from build123d import *

# Parameters (mm, degrees)
BOSS_EXTRUDE1_DEPTH = 19.05
SKETCH3_W           = 5
SKETCH3_H           = 26.05
CUT_EXTRUDE2_DEPTH  = 3
BOSS_EXTRUDE2_DEPTH = 38.1
SKETCH5_R           = 1.5
CUT_EXTRUDE3_DEPTH  = 8.35
FILLET1_R           = 1


with BuildPart() as part:
    # Sketch1 → Boss-Extrude1 (new body, symmetric)
    with BuildSketch(Plane(origin=(0, 0, 0), x_dir=(0, 0, -1), z_dir=(1, 0, 0))):
        Polygon((0, 0), (-2, 0), (-2, 38), (-40, 38), (-40, 40), (0, 40), align=None)
    extrude(amount=BOSS_EXTRUDE1_DEPTH, both=True)

    # Sketch3 → Cut-Extrude2 (cut, through all)
    with BuildSketch(Plane.XY.offset(2)):
        with Locations((2.5, 17.394531681)):
            Rectangle(SKETCH3_W, SKETCH3_H)
        with Locations((-2.5, 17.394531681)):
            Rectangle(SKETCH3_W, SKETCH3_H)
        with BuildLine():
            Line((-9.525, 30.419531681), (-9.525, 20.419531681))
            ThreePointArc((-9.525, 20.419531681), (-8.025, 18.919531681), (-6.525, 20.419531681))
            Line((-6.525, 20.419531681), (-6.525, 30.419531681))
            ThreePointArc((-6.525, 30.419531681), (-8.025, 31.919531681), (-9.525, 30.419531681))
        make_face()
        with BuildLine():
            Line((-9.525, 14.369531681), (-9.525, 4.369531681))
            ThreePointArc((-9.525, 4.369531681), (-8.025, 2.869531681), (-6.525, 4.369531681))
            Line((-6.525, 4.369531681), (-6.525, 14.369531681))
            ThreePointArc((-6.525, 14.369531681), (-8.025, 15.869531681), (-9.525, 14.369531681))
        make_face()
        with BuildLine():
            ThreePointArc((9.525, 20.419531681), (8.025, 18.919531681), (6.525, 20.419531681))
            Line((6.525, 20.419531681), (6.525, 30.419531681))
            ThreePointArc((6.525, 30.419531681), (8.025, 31.919531681), (9.525, 30.419531681))
            Line((9.525, 30.419531681), (9.525, 20.419531681))
        make_face()
        with BuildLine():
            ThreePointArc((9.525, 4.369531681), (8.025, 2.869531681), (6.525, 4.369531681))
            Line((6.525, 4.369531681), (6.525, 14.369531681))
            ThreePointArc((6.525, 14.369531681), (8.025, 15.869531681), (9.525, 14.369531681))
            Line((9.525, 14.369531681), (9.525, 4.369531681))
        make_face()
        Polygon((-15.786412439, 30.942427664), (-19.05, 34.716026675), (-19.05, 0), (-15.786412439, 0), align=None)
        Polygon((15.786412439, 30.942427664), (15.786412439, 0), (19.05, 0), (19.05, 34.716026675), align=None)
    extrude(amount=-CUT_EXTRUDE2_DEPTH, mode=Mode.SUBTRACT)

    # Sketch4 → Boss-Extrude2 (add)
    with BuildSketch(Plane(origin=(19.05, 0, 0), x_dir=(0, 0, -1), z_dir=(1, 0, 0))):
        Polygon((-2, 38), (-29.84, 31.65), (-40, 31.65), (-40, 38), align=None)
    extrude(amount=-BOSS_EXTRUDE2_DEPTH)

    # Sketch5 → Cut-Extrude3 (cut)
    with BuildSketch(Plane(origin=(0, 40, 0), x_dir=(1, 0, 0), z_dir=(0, 1, 0))):
        with Locations((-12.7, -34.92)):
            Circle(SKETCH5_R)
        with Locations((12.7, -34.92)):
            Circle(SKETCH5_R)
    extrude(amount=-CUT_EXTRUDE3_DEPTH, mode=Mode.SUBTRACT)

    # Fillet1
    fillet1_edges = [part.edges().sort_by_distance(p)[0] for p in [
        (0, 38, 2),
        (0, 40, 40),
        (0, 31.65, 29.84),
        (19.05, 35.825, 40),
        (-19.05, 35.825, 40),
        (-19.05, 40, 20),
        (19.05, 40, 20),
    ]]
    fillet(fillet1_edges, radius=FILLET1_R)


solid = part.part
Verification items for the finished model (mm, model axes). A direction names the side the tool comes from. Give positions to 0.01 mm unless a question says otherwise; leave off trailing zeros. Write each loop counter-clockwise with the first axis right and the second up, starting at its lowest first coordinate (ties: lowest second). Pieces come first, ordered by that corner, then holes.
(1) Gauge pin test, flat ends, axial feed: pin 1 (6 mm diameter, centred on x = 9.5, y = 18.5, fed in from +Z); pin 2 (2.5 mm diameter, centred on x = 12.7, z = 34.92, fed in from +Y); pin 3 (0.6 mm diameter, centred on y = 25.5, z = 1.5, fed in from -X); pin 4 (1 mm diameter, centred on y = 7, z = 1.5, fed in from +X). Record the tip position at first contact, or that the pin passes through.
(2) Cross-section at A-A (z = 34.92). Enter the section's corners in (x, y).
(3) Cross-section at D-D (y = 29). Enter the section's corners in (x, z) (3 decimals), plus the area to 3 significant figures.
(4) Material ranges on line 1 (X direction, y = 35, z = 34.92); line 2 (X direction, y = 36, z = 34); line 3 (Z direction, x = -4, y = 31.5), recorded low to high.
(5) Cross-section at C-C (x = 0.5). Enter the section's corners in (y, z).
(6) Cross-section at B-B (y = 18). Enter the section's corners in (x, z).
(7) Access from +Z, -Z, +X, -X, +Y, -Y to the whole of each face (thin tool, end or side, straight path). Record for faces 5 (the face through (8.06, 2.87, 1.01)), 6 (the face through (-7.99, 31.92, 1.01)), 7 (the face through (15.786, 16, 1)), 8 (the face through (17.441, 32.856, 1.014)), 9 (the face through (-0.27, 37.54, 2.39)).
(8) Mould release check, pull along Y, two halves, no side actions. Record for faces 1 (the face through (9, 18, 2)), 2 (the face through (0, 40, 20)), 3 (the face through (-9.525, 25, 1)), 4 (the face through (-5, 17, 1)): +Y half, -Y half, draft (parallel to the pull), parting line (faces both ways), or undercut.
Worked out:
1. pin 1: stops at z = 2
1. pin 2: passes through
1. pin 3: stops at x = -15.79
1. pin 4: stops at x = 15.79
2. outline: (-19.05, 31.65) - (-14.2, 31.65) - (-14.2, 40) - (-18.05, 40) arc R1 ccw to (-19.05, 39) - close; (-11.2, 31.65) - (11.2, 31.65) - (11.2, 40) - (-11.2, 40) - close; (14.2, 31.65) - (19.05, 31.65) - (19.05, 39) arc R1 ccw to (18.05, 40) - (14.2, 40) - close
3. outline: (-15.786, 0) - (-9.525, 0) - (-9.525, 2) - (-15.786, 2) - close; (-6.525, 0) - (-5, 0) - (-5, 2) - (-6.525, 2) - close; (5, 0) - (6.525, 0) - (6.525, 2) - (5, 2) - close; (9.525, 0) - (15.786, 0) - (15.786, 2) - (9.525, 2) - close
3. area: 31.1 mm2
4. line 1: x = -19.05 to -14.2, -11.2 to 11.2, 14.2 to 19.05
4. line 2: x = -19.05 to -13.88, -11.52 to 11.52, 13.88 to 19.05
4. line 3: z = 0 to 2
5. outline: (0, 0) - (4.37, 0) - (4.37, 2) - (0, 2) - close; (30.42, 0) - (40, 0) - (40, 39) arc R1 ccw to (39, 40) - (31.65, 40) - (31.65, 29.95) arc R1 ccw to (31.68, 29.73) - (37.72, 3.22) arc R1 cw to (36.75, 2) - (30.42, 2) - close
6. outline: (-15.79, 0) - (-5, 0) - (-5, 2) - (-15.79, 2) - close; (5, 0) - (15.79, 0) - (15.79, 2) - (5, 2) - close
7. face 5: +Z, -Z
7. face 6: -Z
7. face 7: +Z, -Z, +X, -Y
7. face 8: -Z, +X, -Y
7. face 9: +X, -X, -Y
8. face 1: draft
8. face 2: +Y half
8. face 3: undercut
8. face 4: undercut
